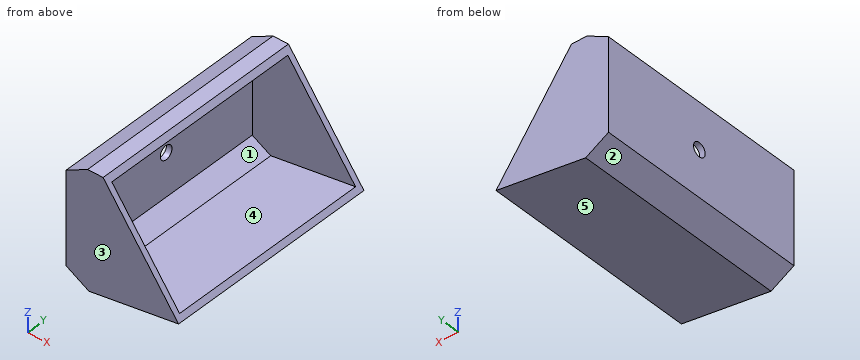
```python
from build123d import *

# Parameters (mm, degrees)
F1_DEPTH = 25.4
F2_DEPTH = 75.184
F3_T     = -2.54
F6_D     = 6.35


with BuildPart() as f1:
    # F0 (on Front) → F1 (new body)
    with BuildSketch(Plane.XZ):
        Polygon((-45.7421503961, 42.3308722675), (-45.7421503961, 0), (-35.1981967688, -6.0472674668), (6.0472679324, 0), (-28.6857560277, 47.6028472185), (-35.8184315264, 47.6028472185), align=None)
    extrude(amount=F1_DEPTH)

    # F2 (add): a face of the model
    f2_faces = [f1.faces().sort_by_distance(p)[0] for p in [
        (-26.6568432389, 0, 17.4826734164),
    ]]
    extrude(f2_faces, amount=F2_DEPTH)

    # F3
    f3_openings = [f1.faces().sort_by_distance(p)[0] for p in [
        (-11.319244, 24.892, 23.801424),
    ]]
    offset(amount=F3_T, openings=f3_openings)

    # F6 (through all)
    with Locations(Plane(origin=(-45.7421503961, 0, 0), x_dir=(0, -1, 0), z_dir=(-1, 0, 0))):
        with Locations((-25.9138997644, 21.2229900062)):
            Hole(F6_D / 2)


solid = f1.part
```
For this review, take the finished solid that the model builds, in its own axes (mm). Face numbers are marked on the shaded views. A direction names the side the tool comes from. Round coordinates to 2 decimals unless told otherwise and drop trailing zeros. Write each loop counter-clockwise with the first axis right and the second up, starting at its lowest first coordinate (ties: lowest second). Pieces come first, ordered by that corner, then holes.
1) Take a section at D-D on x = -37. Give the boundary of the cut face in (y, z), then the cut area to 3 significant figures.
Answer below:
outline: (-25.4, -5.01) - (75.18, -5.01) - (75.18, 46.98) - (-25.4, 46.98) - close; hole (-22.86, -2.09) - (72.64, -2.09) - (72.64, 44.1) - (-22.86, 44.1) - close
area: 818 mm2
2) Take a section at A-A on y = 2.5. Give the boundary of the cut face in (x, z).
Answer below:
outline: (-45.74, 0) - (-35.2, -6.05) - (6.05, 0) - (4.36, 2.32) - (-34.7, -3.41) - (-43.2, 1.47) - (-43.2, 40.8) - (-35.19, 45.06) - (-26.83, 45.06) - (-28.69, 47.6) - (-35.82, 47.6) - (-45.74, 42.33) - close
3) Insertion check: pin 1 Ø6 at (x, y) = (-22.5, 31) entering from +Z; pin 2 Ø12 at (y, z) = (26.5, 22) entering from +X; pin 3 Ø1.5 at (x, y) = (-12.5, 21) entering from -Z; pin 4 Ø5.5 at (y, z) = (25.91, 21.22) entering from +X. Each pin has a flat end and moves straight along its axis. Give the tip position at first contact, or say it passes through.
Answer below:
pin 1: stops at z = -1.18
pin 2: stops at x = -43.2
pin 3: stops at z = -2.83
pin 4: passes through
4) For line 1 along Y through (x, z) = (-23.5, 8); line 2 along X through (y, z) = (40.5, 6); line 3 along Z through (x, y) = (-30, -1), list the stretches that pass through material, from the lowest coordinate up.
Answer below:
line 1: y = -25.4 to -22.86, 72.64 to 75.18
line 2: x = -45.74 to -43.2
line 3: z = -5.29 to -2.72, 45.06 to 47.6
5) Take a section at B-B on z = 28.5. Give the boundary of the cut face in (x, y).
Answer below:
outline: (-45.74, -25.4) - (-14.75, -25.4) - (-14.75, -22.86) - (-43.2, -22.86) - (-43.2, 72.64) - (-14.75, 72.64) - (-14.75, 75.18) - (-45.74, 75.18) - close
6) Take a section at C-C on x = -20. Give the boundary of the cut face in (y, z).
Answer below:
outline: (-25.4, -3.82) - (75.18, -3.82) - (75.18, 35.7) - (72.64, 35.7) - (72.64, -1.25) - (-22.86, -1.25) - (-22.86, 35.7) - (-25.4, 35.7) - close
7) Machinability: for the marked faces 4 and 5, which of the approach directions +Z, -Z, +X, -X, +Y, -Y give a long, thin tool a straight path to every point of the face, cutting with its end or side? Answer none if there is none.
Answer below:
face 4: none
face 5: -Z, +X, +Y, -Y
8) Mouldability with a two-part tool opening along Z and no side actions: class the marked faces 1, 2 and 3 as +Z half, -Z half, draft (parallel to the pull), parting line (faces both ways), or undercut.
Answer below:
face 1: undercut
face 2: -Z half
face 3: draft
